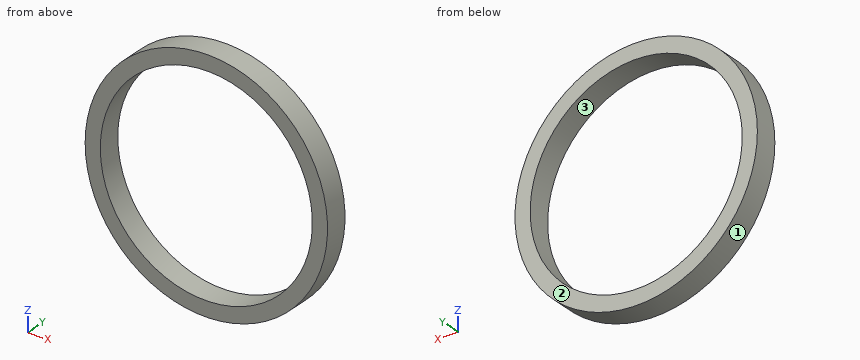
Autodesk Inventor part; units mm, degrees
ref_plane "YZ Plane" through (0, 0, 0) normal (1, 0, 0) x (0, 1, 0)
ref_plane "XZ Plane" through (0, 0, 0) normal (0, 1, 0) x (-1, 0, 0)
ref_plane "XY Plane" through (0, 0, 0) normal (0, 0, 1) x (1, 0, 0)
sketch "Sketch1" plane through (0, 0, 0) normal (0, 1, 0) x (-1, 0, 0)
  circle A0 centre (0, 0) radius 50.8
  circle A1 centre (0, 0) radius 44.45
  dimension "d0" = 88.9
  dimension "d1" = 101.6
extrude "Extrusion1" add sketch "Sketch1" along normal mid plane 10
sketch "Sketch2" plane through (0, 0, 0) normal (0, 1, 0) x (-1, 0, 0)
  circle A0 centre (0, 0) radius 50.8 construction
  line L0 (50.8, 0) -> (44.45, 0) construction
  circle A1 centre (0, 0) radius 44.45 construction
  line L1 (46.125, 3) -> (49.125, 3)
  line L2 (49.125, 3) -> (49.125, -3)
  line L3 (49.125, -3) -> (46.125, -3)
  line L4 (46.125, -3) -> (46.125, 3)
  line L5 (46.125, 3) -> (49.125, -3) construction
  line L6 (49.125, 3) -> (46.125, -3) construction
  line L7 (42.9404, -17.1066) -> (44.7945, -11.4002)
  line L8 (45.7936, -18.0336) -> (42.9404, -17.1066)
  line L9 (47.6477, -12.3273) -> (45.7936, -18.0336)
  line L10 (44.7945, -11.4002) -> (47.6477, -12.3273)
  line L11 (35.5526, -29.5386) -> (39.0793, -24.6845)
  line L12 (37.9796, -31.302) -> (35.5526, -29.5386)
  line L13 (41.5063, -26.4479) -> (37.9796, -31.302)
  line L14 (39.0793, -24.6845) -> (41.5063, -26.4479)
  line L15 (24.6845, -39.0793) -> (29.5386, -35.5526)
  line L16 (26.4479, -41.5063) -> (24.6845, -39.0793)
  line L17 (31.302, -37.9796) -> (26.4479, -41.5063)
  line L18 (29.5386, -35.5526) -> (31.302, -37.9796)
  line L19 (11.4002, -44.7945) -> (17.1066, -42.9404)
  line L20 (12.3273, -47.6477) -> (11.4002, -44.7945)
  line L21 (18.0336, -45.7936) -> (12.3273, -47.6477)
  line L22 (17.1066, -42.9404) -> (18.0336, -45.7936)
  line L23 (-3, -46.125) -> (3, -46.125)
  line L24 (-3, -49.125) -> (-3, -46.125)
  line L25 (3, -49.125) -> (-3, -49.125)
  line L26 (3, -46.125) -> (3, -49.125)
  line L27 (-17.1066, -42.9404) -> (-11.4002, -44.7945)
  line L28 (-18.0336, -45.7936) -> (-17.1066, -42.9404)
  line L29 (-12.3273, -47.6477) -> (-18.0336, -45.7936)
  line L30 (-11.4002, -44.7945) -> (-12.3273, -47.6477)
  line L31 (-29.5386, -35.5526) -> (-24.6845, -39.0793)
  line L32 (-31.302, -37.9796) -> (-29.5386, -35.5526)
  line L33 (-26.4479, -41.5063) -> (-31.302, -37.9796)
  line L34 (-24.6845, -39.0793) -> (-26.4479, -41.5063)
  line L35 (-39.0793, -24.6845) -> (-35.5526, -29.5386)
  line L36 (-41.5063, -26.4479) -> (-39.0793, -24.6845)
  line L37 (-37.9796, -31.302) -> (-41.5063, -26.4479)
  line L38 (-35.5526, -29.5386) -> (-37.9796, -31.302)
  line L39 (-44.7945, -11.4002) -> (-42.9404, -17.1066)
  line L40 (-47.6477, -12.3273) -> (-44.7945, -11.4002)
  line L41 (-45.7936, -18.0336) -> (-47.6477, -12.3273)
  line L42 (-42.9404, -17.1066) -> (-45.7936, -18.0336)
  line L43 (-46.125, 3) -> (-46.125, -3)
  line L44 (-49.125, 3) -> (-46.125, 3)
  line L45 (-49.125, -3) -> (-49.125, 3)
  line L46 (-46.125, -3) -> (-49.125, -3)
  line L47 (-42.9404, 17.1066) -> (-44.7945, 11.4002)
  line L48 (-45.7936, 18.0336) -> (-42.9404, 17.1066)
  line L49 (-47.6477, 12.3273) -> (-45.7936, 18.0336)
  line L50 (-44.7945, 11.4002) -> (-47.6477, 12.3273)
  line L51 (-35.5526, 29.5386) -> (-39.0793, 24.6845)
  line L52 (-37.9796, 31.302) -> (-35.5526, 29.5386)
  line L53 (-41.5063, 26.4479) -> (-37.9796, 31.302)
  line L54 (-39.0793, 24.6845) -> (-41.5063, 26.4479)
  line L55 (-24.6845, 39.0793) -> (-29.5386, 35.5526)
  line L56 (-26.4479, 41.5063) -> (-24.6845, 39.0793)
  line L57 (-31.302, 37.9796) -> (-26.4479, 41.5063)
  line L58 (-29.5386, 35.5526) -> (-31.302, 37.9796)
  line L59 (-11.4002, 44.7945) -> (-17.1066, 42.9404)
  line L60 (-12.3273, 47.6477) -> (-11.4002, 44.7945)
  line L61 (-18.0336, 45.7936) -> (-12.3273, 47.6477)
  line L62 (-17.1066, 42.9404) -> (-18.0336, 45.7936)
  line L63 (3, 46.125) -> (-3, 46.125)
  line L64 (3, 49.125) -> (3, 46.125)
  line L65 (-3, 49.125) -> (3, 49.125)
  line L66 (-3, 46.125) -> (-3, 49.125)
  line L67 (17.1066, 42.9404) -> (11.4002, 44.7945)
  line L68 (18.0336, 45.7936) -> (17.1066, 42.9404)
  line L69 (12.3273, 47.6477) -> (18.0336, 45.7936)
  line L70 (11.4002, 44.7945) -> (12.3273, 47.6477)
  line L71 (29.5386, 35.5526) -> (24.6845, 39.0793)
  line L72 (31.302, 37.9796) -> (29.5386, 35.5526)
  line L73 (26.4479, 41.5063) -> (31.302, 37.9796)
  line L74 (24.6845, 39.0793) -> (26.4479, 41.5063)
  line L75 (39.0793, 24.6845) -> (35.5526, 29.5386)
  line L76 (41.5063, 26.4479) -> (39.0793, 24.6845)
  line L77 (37.9796, 31.302) -> (41.5063, 26.4479)
  line L78 (35.5526, 29.5386) -> (37.9796, 31.302)
  line L79 (44.7945, 11.4002) -> (42.9404, 17.1066)
  line L80 (47.6477, 12.3273) -> (44.7945, 11.4002)
  line L81 (45.7936, 18.0336) -> (47.6477, 12.3273)
  line L82 (42.9404, 17.1066) -> (45.7936, 18.0336)
  point P0 (47.625, 0)
  dimension "d4" = 3
  dimension "d5" = 6
  dimension "d8" = 360
extrude "Extrusion2" cut sketch "Sketch2" along normal mid plane 6
properties part number "ring_ABS"
Geometry check sheet. Reference: the model listing, model coordinates, mm. Face numbers are marked on the shaded views. Give positions to 0.01 mm unless a question says otherwise; leave off trailing zeros. Loops run counter-clockwise (first coordinate to the right, second up) from the corner with the lowest first, then second, coordinate; pieces in that order, holes last. Notation, with made-up numbers: M 88,-28.75 L 120,-28.75 A29 ccw 120,4.25 Z; hole C 52.5,27.25 d6. An arc over 180 degrees is marked long. Answer as a JSON object with one key per item and string values. Group by question number.
Item 1: Sectioned sample at B-B on x = 0. Record the boundary of the cut face in (y, z) (3 decimals).
Item 2: Gauge pin test, flat ends, axial feed: pin 1 (2.5 mm diameter, centred on y = -1, z = -48, fed in from +X); pin 2 (5 mm diameter, centred on y = 3, z = -31, fed in from +X); pin 3 (3 mm diameter, centred on y = 2.5, z = -25, fed in from -X); pin 4 (3 mm diameter, centred on y = 0, z = -1, fed in from -X). Record the tip position at first contact, or that the pin passes through.
Item 3: Material ranges on L1, parallel to Z at x = 0, y = 2.25 (3 decimals); L2, parallel to X at y = -2.5, z = 25.5; L3, parallel to X at y = 2.25, z = 36.5, recorded low to high.
Item 4: Sectioned sample at C-C on x = -21.5. Record the boundary of the cut face in (y, z), plus the area to 3 significant figures.
Item 5: Mould release check, pull along X, two halves, no side actions. Record for the marked faces 1, 2 and 3: pulls with the +X half, pulls with the -X half, needs draft (parallel to the pull), parting line crosses it, or undercut.
Item 6: Sectioned sample at A-A on z = 0. Record the boundary of the cut face in (x, y) (3 decimals).
Findings below:
{
 "1": {"outline": "M -5,-50.8 L 5,-50.8 L 5,-44.45 L -5,-44.45 Z; M -5,44.45 L 5,44.45 L 5,50.8 L -5,50.8 Z; hole M -3,-49.125 L 3,-49.125 L 3,-46.125 L -3,-46.125 Z; hole M -3,46.125 L 3,46.125 L 3,49.125 L -3,49.125 Z"},
 "2": {"pin 1": "x = 19.88", "pin 2": "x = 42.05", "pin 3": "x = -45.04", "pin 4": "x = -50.8"},
 "3": {"L1": "-50.8 to -49.125, -46.125 to -44.45, 44.45 to 46.125, 49.125 to 50.8", "L2": "-43.94 to -40.2, -38.49 to -36.41, 36.41 to 38.49, 40.2 to 43.94", "L3": "-35.33 to -30.23, -28.23 to -25.37, 25.37 to 28.23, 30.23 to 35.33"},
 "4": {"outline": "M -5,-46.03 L 5,-46.03 L 5,-38.9 L -5,-38.9 Z; M -5,38.9 L 5,38.9 L 5,46.03 L -5,46.03 Z", "area": "142 mm2"},
 "5": {"face 1": "parting line crosses it", "face 2": "needs draft", "face 3": "undercut"},
 "6": {"outline": "M -50.8,-5 L -44.45,-5 L -44.45,5 L -50.8,5 Z; M 44.45,-5 L 50.8,-5 L 50.8,5 L 44.45,5 Z; hole M -49.125,-3 L -46.125,-3 L -46.125,3 L -49.125,3 Z; hole M 46.125,-3 L 49.125,-3 L 49.125,3 L 46.125,3 Z"}
}
